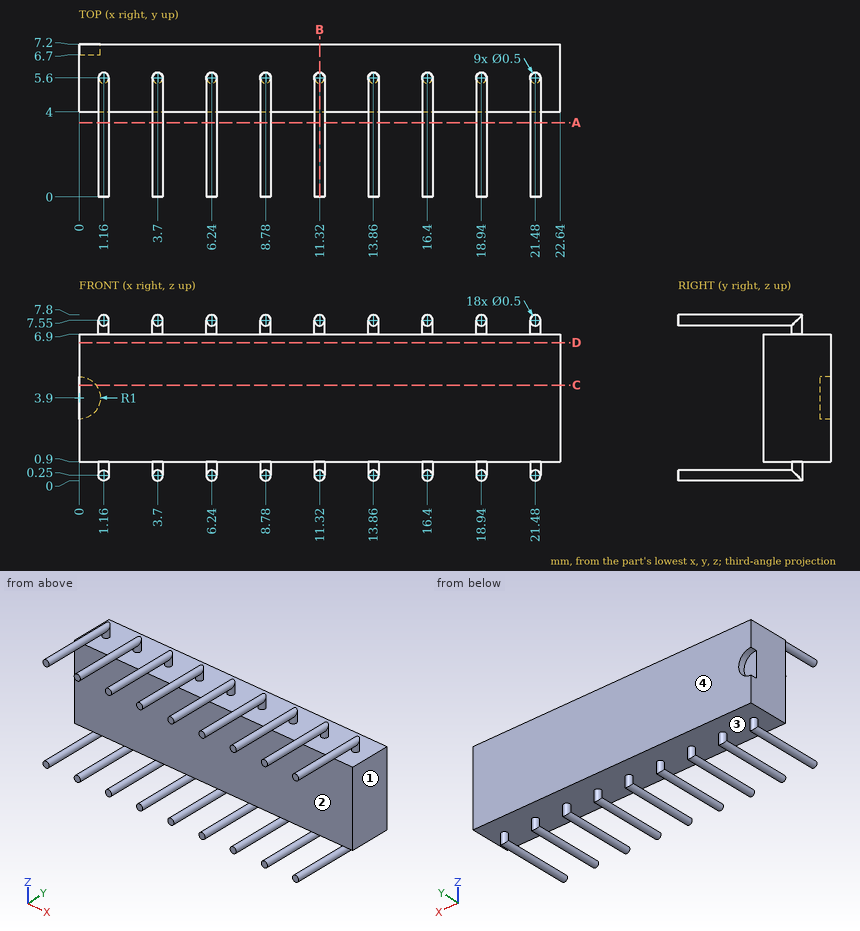
Part print with two shaded views. Sizes in mm from the minimum x, y, z corner. A direction names the side the tool comes from. Round coordinates to 2 decimals unless told otherwise and drop trailing zeros. Order: outer loops, then holes, each group sorted by start corner. A loop starts at its lowest first (then second) coordinate and runs counter-clockwise, first axis right, second up. Notation, with made-up numbers: (60.25, 42) - (74.25, 42) arc R21 ccw to (74.25, 77) - close; hole circle Ø9 at (86.25, -31.5). An arc over 180 degrees is marked (long way). Return JSON: item names as keys, results as strings.
(1) Cut at C-C (z = 4.5). Give the cut face in (x, y), then the cut area to 3 significant figures.
Answer key:
{"outline": "(0, 4) - (22.64, 4) - (22.64, 7.2) - (0.8, 7.2) - (0.8, 6.7) - (0, 6.7) - close", "area": "72.0 mm^2"}
(2) Cut at B-B (x = 11.32). Give the cut face in (y, z).
Answer key:
{"outline": "(0, 0) - (5.85, 0) - (5.85, 0.9) - (7.2, 0.9) - (7.2, 6.9) - (5.85, 6.9) - (5.85, 7.8) - (0, 7.8) - (0, 7.3) - (5.35, 7.3) - (5.35, 6.9) - (4, 6.9) - (4, 0.9) - (5.35, 0.9) - (5.35, 0.5) - (0, 0.5) - close"}
(3) Pull direction Z, two halves, no side cores. Call the marked faces 3 and 4: +Z half, -Z half, draft (parallel to the pull), parting line (faces both ways), or undercut.
Answer key:
{"face 3": "undercut", "face 4": "draft"}
(4) Tool access for the marked faces 1 and 2: list every direction of +Z, -Z, +X, -X, +Y, -Y with a clear straight run to the whole face (end or side of a thin tool).
Answer key:
{"face 1": "+Z, -Z, +X, +Y, -Y", "face 2": "+X, -X, -Y"}
(5) Cut at A-A (y = 3.5). State how many separate pieces and enclosed holes the cut face has, then the cut area to 3 significant figures.
Answer key:
{"separate pieces": "18", "enclosed holes": "0", "area": "3.53 mm^2"}
(6) Cut at D-D (z = 6.5). Give the cut face in (x, y).
Answer key:
{"outline": "(0, 4) - (22.64, 4) - (22.64, 7.2) - (0, 7.2) - close"}
(7) Pin check, flat tips, straight feed: pin 1 Ø0.5 at (x, z) = (0.5, 4) entering from +Y; pin 2 Ø3 at (x, z) = (6, 5) entering from -Y. Stop position of each tip, or through.
Answer key:
{"pin 1": "stops at y = 6.7", "pin 2": "stops at y = 4"}
(8) Wall check: probe 1 along Z at (x, y) = (6.25, 0.5); probe 2 along Z at (x, y) = (15, 4.5); probe 3 along Y at (x, z) = (21.25, 5.5). Give the ranges that are in metal, low to high. Write a range as from..to.
Answer key:
{"probe 1": "z = 0..0.5, 7.3..7.8", "probe 2": "z = 0.9..6.9", "probe 3": "y = 4..7.2"}
